from build123d import *

# Parameters (mm, degrees)
F0_W     = 51.6446605325
F0_H     = 48.6768968403
F1_DEPTH = 63.5
F3_DEPTH = 63.5
F4_R     = 24.3384484202
F6_DEPTH = 25.399999693


# Not quite as in the source:
# - the program builds the solid bodies; features that only make, move or delete a surface that nothing else refers to are left out


with BuildPart() as f1:
    # F0 (on Right) → F1 (new body)
    with BuildSketch(Plane.YZ):
        with Locations((25.8223302662, -24.3384484202)):
            Rectangle(F0_W, F0_H)
    extrude(amount=F1_DEPTH)

    # F2 (on face) → F3 (join)
    with BuildSketch(Plane.YZ.offset(63.5)):
        with BuildLine():
            ThreePointArc((25.8223302662, -48.6768968403), (43.0322121877, -41.5483303416), (50.1607786864, -24.3384484202))
            ThreePointArc((50.1607786864, -24.3384484202), (43.0322121877, -7.1285664987), (25.8223302662, 0))
            ThreePointArc((25.8223302662, 0), (1.4838818461, -24.3384484202), (25.8223302662, -48.6768968403))
        make_face()
    extrude(amount=F3_DEPTH)

    # F4 (on face) + F5 (on face) → F6 (cut)
    with BuildSketch(Plane.YZ.offset(127)):
        with Locations((25.8223302662, -24.3384484202)):
            Circle(F4_R)
    with BuildSketch(Plane.YZ.offset(127)):
        with BuildLine():
            add(Edge.make_bspline(
                [(24.2070443928, -3.5950578749), (13.7185256549, -3.5950578749), (18.9627850239, -34.8861049861), (24.2070443928, -66.1771520972), (29.4513037618, -34.8861049861), (34.6955631307, -3.5950578749), (24.2070443928, -3.5950578749)],
                knots=[0, 0, 0, 2.0943951024, 2.0943951024, 4.1887902048, 4.1887902048, 6.2831853072, 6.2831853072, 6.2831853072], degree=2, weights=[1, 0.5, 1, 0.5, 1, 0.5, 1]))
        make_face()
    extrude(amount=F6_DEPTH, mode=Mode.SUBTRACT)


solid = f1.part
Design review of the part built by this model. Coordinates are the model's own, in mm. A direction names the side the tool comes from. Give positions to 0.01 mm unless a question says otherwise; leave off trailing zeros. Loops run counter-clockwise (first coordinate to the right, second up) from the corner with the lowest first, then second, coordinate; pieces in that order, holes last. Notation, with made-up numbers: (-34.75, -35.75) - (15.25, -35.75) arc R15 cw to (15.25, -26.75) - close; hole circle Ø2 at (2, 9). An arc over 180 degrees is marked (long way). Use CSV: the item, a comma, the result in double quotes. Start each with the question number.
1. Add section A-A (z = -8). State the section outline as (x, y) points.
2. Machinability: for faces 1 (the cylindrical face through (94.806, 18.512, -1.124)), 2 (the flat face through (63.5, 1, -24)), 3 (the flat face through (63.5, 50.1, -20.6)), which of the approach directions +Z, -Z, +X, -X, +Y, -Y give a long, thin tool a straight path to every point of the face, cutting with its end or side? Answer none if there is none.
3. Wall thickness on L1, parallel to X at y = 2, z = -5; L2, parallel to Z at x = 106.5, y = 37; L3, parallel to Y at x = 111, z = -8: over which ranges is each line inside the solid? List them lowest first.
4. Add section B-B (y = 48.5). State the section outline as (x, z) points.
5. Insertion check: P1, Ø3, axis at x = 77, z = -18, coming from the -Y side; P2, Ø1.5, axis at x = 78, z = -6.5, coming from the -Y side. Each pin has a flat end and moves straight along its axis. Give the tip position at first contact, or say it passes through.
6. Add section C-C (x = 119). State the section outline as (y, z) points.
Results found:
1,outline,"(0, 0) - (63.5, 0) - (63.5, 7.78) - (127, 7.78) - (127, 43.86) - (63.5, 43.86) - (63.5, 51.64) - (0, 51.64) - close"
2,face 1,"+X"
2,face 2,"+X, -Y"
2,face 3,"+X, +Y"
3,L1,"x = 0 to 63.5"
3,L2,"z = -45.96 to -2.72"
3,L3,"y = 7.78 to 43.86"
4,outline,"(0, -48.68) - (63.5, -48.68) - (63.5, -33.17) - (127, -33.17) - (127, -15.5) - (63.5, -15.5) - (63.5, 0) - (0, 0) - close"
5,P1,"stops at y = 1.97"
5,P2,"stops at y = 8.49"
6,outline,"circle Ø48.68 at (25.82, -24.34)"
